The listing builds one solid part. Answer for the finished solid, in the listing's coordinates (mm). Face numbers are marked on the shaded views. A direction names the side the tool comes from. Give positions to 0.01 mm unless a question says otherwise; leave off trailing zeros. Loops run counter-clockwise (first coordinate to the right, second up) from the corner with the lowest first, then second, coordinate; pieces in that order, holes last. Notation, with made-up numbers: (43.5, 25.5) - (54.5, 25.5) arc R29 cw to (54.5, 61.5) - close; hole circle Ø5 at (69.5, -26.75). An arc over 180 degrees is marked (long way). Answer in a Markdown table with one row per item. Add a question column.
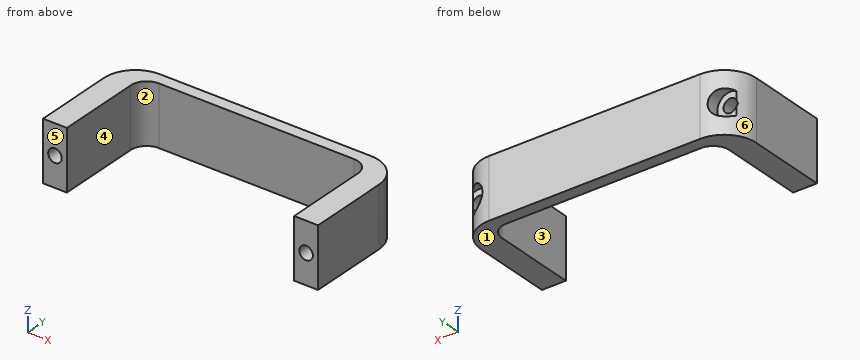
```python
from build123d import *

# Parameters (mm, degrees)
P_IDAT_VYSUNUT_M1_DEPTH                          = 15
V_LCOV_ZAHLOUBEN_PRO_M3_ROUBY_S_VNIT_D           = 3.4
V_LCOV_ZAHLOUBEN_PRO_M3_ROUBY_S_VNIT_CBORE_D     = 6.5
V_LCOV_ZAHLOUBEN_PRO_M3_ROUBY_S_VNIT_CBORE_DEPTH = 3.4


with BuildPart() as part:
    # Skica1 → Přidat vysunutím1 (new body)
    with BuildSketch(Plane.XY):
        with BuildLine():
            Line((-23.771796173, 0), (29.228203827, 0))
            ThreePointArc((29.228203827, 0), (34.885058077, -2.343145751), (37.228203827, -8))
            Line((37.228203827, -8), (37.228203827, -28))
            Line((37.228203827, -28), (31.228203827, -28))
            Line((31.228203827, -28), (31.228203827, -7))
            ThreePointArc((31.228203827, -7), (30.056630952, -4.171572875), (27.228203827, -3))
            Line((27.228203827, -3), (-21.771796173, -3))
            ThreePointArc((-21.771796173, -3), (-24.600223298, -4.171572875), (-25.771796173, -7))
            Line((-25.771796173, -7), (-25.771796173, -28))
            Line((-25.771796173, -28), (-31.771796173, -28))
            Line((-31.771796173, -28), (-31.771796173, -8))
            ThreePointArc((-31.771796173, -8), (-29.428650422, -2.343145751), (-23.771796173, 0))
        make_face()
    extrude(amount=P_IDAT_VYSUNUT_M1_DEPTH)

    # Válcové zahloubení pro M3 šrouby s vnitřním šestihranem1 (through all)
    with Locations(Plane(origin=(0, 0, 0), x_dir=(1, 0, 0), z_dir=(0, 1, 0))):
        with Locations((-28.771796173, -7.5), (34.228203827, -7.5)):
            CounterBoreHole(V_LCOV_ZAHLOUBEN_PRO_M3_ROUBY_S_VNIT_D / 2, V_LCOV_ZAHLOUBEN_PRO_M3_ROUBY_S_VNIT_CBORE_D / 2, V_LCOV_ZAHLOUBEN_PRO_M3_ROUBY_S_VNIT_CBORE_DEPTH)


solid = part.part
```
(1) A tool of negligible diameter and unlimited length cuts with its end or side. For the marked faces 1 and 2, from which of +Z, -Z, +X, -X, +Y, -Y can it reach the whole face along a straight path? Write none if from no direction.
(2) A cutting plane is placed at C-C on x = 6. Determine the outline of the cut face in (y, z), plus the area to 3 significant figures.
(3) A cutting plane is placed at B-B on z = 1.25. Determine the outline of the cut face in (x, y).
(4) Find the intervals of material crossed by line 1 along X through (y, z) = (-16, 7.5); line 2 along X through (y, z) = (-24.75, 9); line 3 along X through (y, z) = (-7.5, 5.75), in increasing order. Write a range as [from, to].
(5) A cutting plane is placed at A-A on y = -12.25. Determine the outline of the cut face in (x, z), plus the area to 3 significant figures.
(6) The mould has two halves that part along X. Classify the marked faces 3, 4, 5 and 6: pulls with the +X half, pulls with the -X half, needs draft (parallel to the pull), parting line crosses it, or undercut.
(7) A cutting plane is placed at D-D on z = 7.5. Determine the outline of the cut face in (x, y), plus the area to 3 significant figures.
(8) Given pin 1 Ø4 at (x, z) = (34.5, 7.5) entering from +Y; pin 2 Ø5 at (x, z) = (8, 10) entering from -Y, each flat-ended and moving along its own axis, determine where each tip first touches the part or whether it passes through.
Evaluation:
| question | item | result |
|---|---|---|
| 1 | face 1 | -Z, +X, -X, +Y, -Y |
| 1 | face 2 | +Z, -Z, -Y |
| 2 | outline | (-3, 0) - (0, 0) - (0, 15) - (-3, 15) - close |
| 2 | area | 45.0 mm² |
| 3 | outline | (-31.77, -28) - (-25.77, -28) - (-25.77, -7) arc R4 cw to (-21.77, -3) - (27.23, -3) arc R4 cw to (31.23, -7) - (31.23, -28) - (37.23, -28) - (37.23, -8) arc R8 ccw to (29.23, 0) - (-23.77, 0) arc R8 ccw to (-31.77, -8) - close |
| 4 | line 1 | x = [-31.77, -30.47], [-27.07, -25.77], [31.23, 32.53], [35.93, 37.23] |
| 4 | line 2 | x = [-31.77, -29.57], [-27.97, -25.77], [31.23, 33.43], [35.03, 37.23] |
| 4 | line 3 | x = [-31.76, -25.77], [31.23, 37.21] |
| 5 | outline | (-31.77, 0) - (-25.77, 0) - (-25.77, 15) - (-31.77, 15) - close; (31.23, 0) - (37.23, 0) - (37.23, 15) - (31.23, 15) - close; hole circle Ø3.4 at (-28.77, 7.5); hole circle Ø3.4 at (34.23, 7.5) |
| 5 | area | 162 mm² |
| 6 | face 3 | undercut |
| 6 | face 4 | undercut |
| 6 | face 5 | needs draft |
| 6 | face 6 | pulls with the -X half |
| 7 | outline | (-31.77, -28) - (-30.47, -28) - (-30.47, -3.63) arc R8 ccw to (-31.77, -8) - close; (-27.07, -28) - (-25.77, -28) - (-25.77, -7) arc R4 cw to (-21.77, -3) - (27.23, -3) arc R4 cw to (31.23, -7) - (31.23, -28) - (32.53, -28) - (32.53, -3.4) - (30.98, -3.4) - (30.98, -0.19) arc R8 ccw to (29.23, 0) - (-23.77, 0) arc R8 ccw to (-25.52, -0.19) - (-25.52, -3.4) - (-27.07, -3.4) - close; (35.93, -28) - (37.23, -28) - (37.23, -8) arc R8 ccw to (35.93, -3.63) - close |
| 7 | area | 300 mm² |
| 8 | pin 1 | stops at y = -3.4 |
| 8 | pin 2 | stops at y = -3 |
